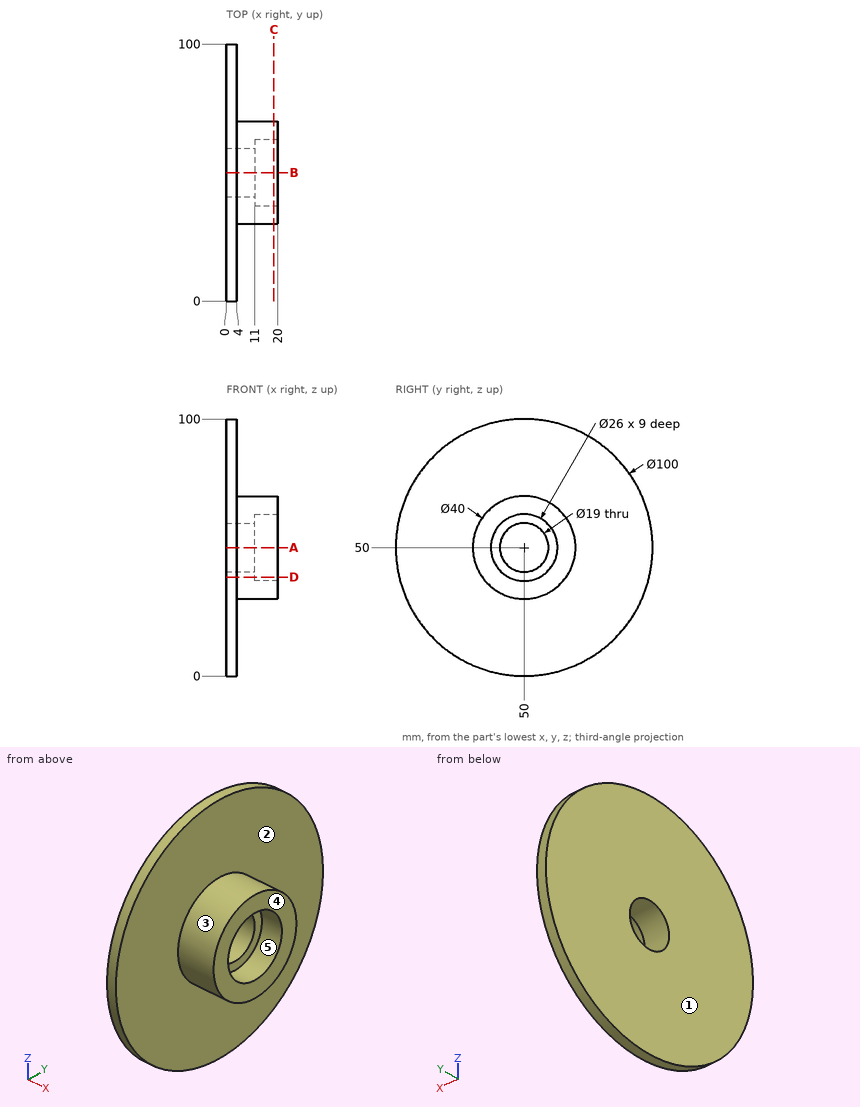
Study the drawing (mm; zero at the part's minimum x, y, z) and answer. A direction names the side the tool comes from. Coordinates: 2 decimals unless noted, no trailing zeros. Write each loop counter-clockwise with the first axis right and the second up, starting at its lowest first coordinate (ties: lowest second). Pieces come first, ordered by that corner, then holes. Notation, with made-up numbers: (11, 11.25) - (52, 11.25) arc R28 cw to (52, 32.25) - close; hole circle Ø8 at (20, -33.5). An arc over 180 degrees is marked (long way). Answer as a JSON object with one key per item and string values. Group by question number.
1. Consider L1, parallel to Y at x = 17.75, z = 59; L2, parallel to X at y = 83, z = 69; L3, parallel to Z at x = 6, y = 44.5. Determine where each line is inside the solid, lowest interval first. Write a range as [from, to].
2. Which of the six approach directions +Z, -Z, +X, -X, +Y, -Y give full straight-line access (tool end or side, diameter ignored) to the marked faces 1 and 2?
3. A cutting plane is placed at A-A (z = 50). Determine the outline of the cut face in (x, y).
4. A cutting plane is placed at D-D (z = 38.5). Determine the outline of the cut face in (x, y), plus the area to 3 significant figures.
5. Each of these flat-tipped pins is pushed along its axis until it touches: P1, Ø12, axis at x = 14, y = 47, coming from the -Z side; P2, Ø8, axis at x = 6.5, y = 83, coming from the +Z side; P3, Ø10, axis at x = 11.5, y = 28, coming from the -Z side. Where does it stop, or does it pass through?
6. A cutting plane is placed at C-C (x = 18.5). Determine the outline of the cut face in (y, z), plus the area to 3 significant figures.
7. The mould has two halves that part along Y. Classify the marked faces 3, 4 and 5: +Y half, -Y half, draft (parallel to the pull), parting line (faces both ways), or undercut.
Worked out:
{
 "1": {"L1": "y = [32.14, 40.62], [59.38, 67.86]", "L2": "x = [0, 4]", "L3": "z = [30.77, 42.25], [57.75, 69.23]"},
 "2": {"face 1": "+Z, -Z, -X, +Y, -Y", "face 2": "+X"},
 "3": {"outline": "(0, 0) - (4, 0) - (4, 30) - (20, 30) - (20, 37) - (11, 37) - (11, 40.5) - (0, 40.5) - close; (0, 59.5) - (11, 59.5) - (11, 63) - (20, 63) - (20, 70) - (4, 70) - (4, 100) - (0, 100) - close"},
 "4": {"outline": "(0, 1.34) - (4, 1.34) - (4, 33.64) - (20, 33.64) - (20, 43.94) - (11, 43.94) - (11, 56.06) - (20, 56.06) - (20, 66.36) - (4, 66.36) - (4, 98.66) - (0, 98.66) - close", "area": "804 mm²"},
 "5": {"P1": "stops at z = 30", "P2": "stops at z = 90.09", "P3": "stops at z = 39.46"},
 "6": {"outline": "circle Ø40 at (50, 50); hole circle Ø26 at (50, 50)", "area": "726 mm²"},
 "7": {"face 3": "parting line", "face 4": "draft", "face 5": "undercut"}
}
